from build123d import *

# Parameters (mm, degrees)
F1_DEPTH  = 15
F2_R      = 2
F3_DEPTH  = 7.5
F4_ANGLE  = 90
F5_R      = 4.5
F6_R      = 2
F10_R     = 2
F11_DEPTH = 5


# Not quite as in the source:
# - a pattern or mirror of a feature is missing from the dataset's text; its kind, count and spacing are read off the source's solid


with BuildPart() as f1:
    # F0 (on Right) → F1 (new body)
    with BuildSketch(Plane.YZ):
        with BuildLine():
            ThreePointArc((-8.7152049129, 10.9565141959), (6.0822336037, 12.6097753505), (14, 0))
            ThreePointArc((14, 0), (6.0822336037, -12.6097753505), (-8.7152049129, -10.9565141959))
            Line((-8.7152049129, -10.9565141959), (-12.2675540951, -14.5088633781))
            ThreePointArc((-12.2675540951, -14.5088633781), (-0.4919673203, -18.993629673), (11.5, -15.1244834623))
            ThreePointArc((11.5, -15.1244834623), (17.0220445305, -8.4409715081), (19, 0))
            ThreePointArc((19, 0), (17.0220445305, 8.4409715081), (11.5, 15.1244834623))
            ThreePointArc((11.5, 15.1244834623), (-0.4919673203, 18.993629673), (-12.2675540951, 14.5088633781))
            Line((-12.2675540951, 14.5088633781), (-8.7152049129, 10.9565141959))
        make_face()
        with BuildLine():
            Line((11.5, 35), (11.5, 15.1244834623))
            ThreePointArc((11.5, 15.1244834623), (17.0220445305, 8.4409715081), (19, 0))
            Line((19, 0), (19, 35))
            Line((19, 35), (11.5, 35))
        make_face()
        with BuildLine():
            ThreePointArc((19, 0), (17.0220445305, -8.4409715081), (11.5, -15.1244834623))
            Line((11.5, -15.1244834623), (11.5, -35))
            Line((11.5, -35), (19, -35))
            Line((19, -35), (19, 0))
        make_face()
    extrude(amount=F1_DEPTH)

    # F2 (on face) → F3 (cut, through all)
    with BuildSketch(Plane.XZ.offset(-11.5)):
        with Locations((7.5, 25.0622417311)):
            Circle(F2_R)
        with Locations((7.5, -25.0622417311)):
            Circle(F2_R)
    extrude(amount=-F3_DEPTH, mode=Mode.SUBTRACT)


with BuildPart() as f1_1:
    # F4: moved
    add(f1.part.rotate(Axis((0, -7, 0), (0, -1, 0)), F4_ANGLE))

    # F5
    f5_edges = [f1_1.edges().sort_by_distance(p)[0] for p in [
        (-15.124483, 11.5, 7.5),
        (15.124483, 11.5, 7.5),
    ]]
    fillet(f5_edges, radius=F5_R)

    # F6
    f6_edges = [f1_1.edges().sort_by_distance(p)[0] for p in [
        (10.956514, -8.715205, 7.5),
        (-10.956514, -8.715205, 7.5),
        (-14.508863, -12.267554, 7.5),
        (14.508863, -12.267554, 7.5),
    ]]
    fillet(f6_edges, radius=F6_R)

    # F10 (on line) → F11 (join)
    with BuildSketch(Plane(origin=(16.2175144213, -6.7175144213, 0), x_dir=(-0.3826834324, -0.9238795325, 0), z_dir=(-0.9238795325, 0.3826834324, 0))):
        with Locations((-1.0217712261, 7.4956147)):
            Circle(F10_R)
    f11 = extrude(amount=-F11_DEPTH)

    # F11_copies: F11 across plane
    add(f11.mirror(Plane(origin=(0, 0, 0), x_dir=(0, 0, -1), z_dir=(-1, 0, 0))))


solid = f1_1.part
Verification items for the finished model (mm, model axes). A direction names the side the tool comes from. Give positions to 0.01 mm unless a question says otherwise; leave off trailing zeros. Write each loop counter-clockwise with the first axis right and the second up, starting at its lowest first coordinate (ties: lowest second). Pieces come first, ordered by that corner, then holes. Notation, with made-up numbers: M 53.5,5 L 107.5,5 A32 cw 107.5,32 Z; hole C -31.5,-30.75 d11. An arc over 180 degrees is marked long. Write item = value, one per line.
(1) Sectioned sample at A-A (y = -1). Record the cut outline in (x, z), then the cut area to 3 significant figures.
Found:
outline = M -18.97,0 L -13.96,0 L -13.96,15 L -18.97,15 Z; M 13.96,0 L 18.97,0 L 18.97,15 L 13.96,15 Z
area = 150 mm2
(2) Access from +Z, -Z, +X, -X, +Y, -Y to the whole of each face (thin tool, end or side, straight path). Record for faces 1 (the face through (0, 17, 0)), 2 (the face through (29, 11.5, 7)), 3 (the face through (11.576, -8.735, 7.605)).
Found:
face_1 = -Z, +X, -X, +Y, -Y
face_2 = +Z, -Z, +X, -Y
face_3 = +Z, -Z
(3) Sectioned sample at C-C (z = 3.5). Record the cut outline in (x, y).
Found:
outline = M -35,11.5 L -22.43,11.5 A4.5 cw -18.14,5.66 A19 ccw -15.97,-10.3 A2 ccw -12.87,-10.63 L -12.15,-9.91 A2 ccw -11.87,-7.43 A14 cw long 11.87,-7.43 A2 ccw 12.15,-9.91 L 12.87,-10.63 A2 ccw 15.97,-10.3 A19 ccw 18.14,5.66 A4.5 cw 22.43,11.5 L 35,11.5 L 35,19 L -35,19 Z
(4) Draft check along Y on faces 4 (the face through (-18.774, 9.619, 7.605)), 5 (the face through (-29, 11.5, 7)), 6 (the face through (-23.11, 15.2, 7.07)). Enter one of: released by +Y, released by -Y, zero draft, split by the parting line, or undercut.
Found:
face_4 = undercut
face_5 = released by -Y
face_6 = zero draft
(5) Sectioned sample at D-D (x = 4). Record the cut outline in (y, z).
Found:
outline = M 13.42,0 L 19,0 L 19,15 L 13.42,15 Z
(6) Go/stop test with flat-tipped pins: pin 1 Ø1 at (x, z) = (-7, 12.5) entering from -Y; pin 2 Ø6.5 at (x, z) = (-30, 9) entering from -Y; pin 3 Ø3.5 at (x, z) = (-25.06, 7.5) entering from +Y; pin 4 Ø3 at (y, z) = (-6.5, 12.5) entering from +X. Record where each tip stops, or that it passes through.
Found:
pin_1 = 11.82
pin_2 = 11.5
pin_3 = through
pin_4 = 18.33
(7) Sectioned sample at B-B (y = 16). Record the cut outline in (x, z).
Found:
outline = M -35,0 L 35,0 L 35,15 L -35,15 Z; hole C -25.06,7.5 d4; hole C 25.06,7.5 d4
(8) Material ranges on line 1 (X direction, y = 14.75, z = 7.5); line 2 (Y direction, x = 14.5, z = 10.5); line 3 (X direction, y = 9.5, z = 9.5), recorded low to high.
Found:
line_1 = -35 to -27.06, -23.06 to 23.06, 27.06 to 35
line_2 = -11.2 to 19
line_3 = -18.69 to -10.28, 10.28 to 18.69
